Source: CAD feature listing. Evaluate the final solid. Frame: model axes, mm. Coordinates: 2 decimals unless noted, no trailing zeros. Order: outer loops, then holes, each group sorted by start corner. A loop starts at its lowest first (then second) coordinate and runs counter-clockwise, first axis right, second up.
Item 1: Section A-A on z = 0. Return the cut outline in (x, y), then the cut area to 3 significant figures.
Item 2: Ray query, line 1 (Y direction, x = 132.7, z = 0); line 2 (Z direction, x = 134.5, y = 16.25); line 3 (Z direction, x = 133.85, y = -21.1). Return the intervals inside material, ascending.
Item 3: Mould query, pull axis Y, two halves, no side actions, for faces 1 (the flat face through (131.7, 20, -20)), 2 (the cylindrical face through (133.672, -30.864, 0.215)), 3 (the cylindrical face through (133.73, -45.61, -5.99)). Classes: released by +Y, released by -Y, zero draft, split by the parting line, or undercut.
Item 4: Section B-B on y = 0. Return the cut outline in (x, z).
Item 5: Section C-C on x = 133.2. Return the cut outline in (y, z), then the cut area to 3 significant figures.
Item 6: Contact query for flat-ended pins moving along their axis: P1, Ø2.5, axis at y = 16.25, z = -28.15, coming from the -X side; P2, Ø1, axis at x = 132, y = 7, coming from the -Z side; P3, Ø2, axis at x = 132, z = -19, coming from the -Y side; P4, Ø1.5, axis at x = 133.5, z = -9, coming from the +Y side. Output: stop coordinate, or through.
Item 7: Section D-D on y = -21.1. Return the cut outline in (x, z), then the cut area to 3 significant figures.
from build123d import *

# Parameters (mm, degrees)
AXIAL_PROFILE_MM_W     = 4
AXIAL_PROFILE_MM_H     = 19
AXIAL_HOLES_DEPTH      = 151.487507787
AXIAL_HOLES_DEPTH_BACK = 151.487507787
SKETCH2_R              = 1.65


with BuildPart() as part:
    # Axial profile (mm) → Full revolution (revolve)
    with BuildSketch(Plane.XY, mode=Mode.PRIVATE) as full_revolution_sk:
        with Locations((133.7, 36.5)):
            Rectangle(AXIAL_PROFILE_MM_W, AXIAL_PROFILE_MM_H)
    revolve(full_revolution_sk.sketch.rotate(Axis((-110, 0, 0), (1, 0, 0)), 90), axis=Axis((-110, 0, 0), (1, 0, 0)))

    # Sketch2 → Axial holes (cut, two sides: drawn at the far end of the back side and taken through both)
    with BuildSketch(Plane(origin=(0, 0, 0), x_dir=(0, 0, -1), z_dir=(1, 0, 0)).offset(-AXIAL_HOLES_DEPTH_BACK)):
        with Locations((0, 42.2)):
            Circle(SKETCH2_R)
        with Locations((-36.54627204, -21.1)):
            Circle(SKETCH2_R)
        with Locations((36.54627204, -21.1)):
            Circle(SKETCH2_R)
        with Locations((-28.145825623, 16.25)):
            Circle(SKETCH2_R)
        with Locations((0, -32.5)):
            Circle(SKETCH2_R)
        with Locations((28.145825623, 16.25)):
            Circle(SKETCH2_R)
    extrude(amount=AXIAL_HOLES_DEPTH + AXIAL_HOLES_DEPTH_BACK, mode=Mode.SUBTRACT)


solid = part.part
Answer list:
1. outline: (131.7, -46) - (135.7, -46) - (135.7, -34.15) - (131.7, -34.15) - close; (131.7, -30.85) - (135.7, -30.85) - (135.7, -27) - (131.7, -27) - close; (131.7, 27) - (135.7, 27) - (135.7, 40.55) - (131.7, 40.55) - close; (131.7, 43.85) - (135.7, 43.85) - (135.7, 46) - (131.7, 46) - close
1. area: 126 mm2
2. line 1: y = -46 to -34.15, -30.85 to -27, 27 to 40.55, 43.85 to 46
2. line 2: z = -43.03 to -29.8, -26.5 to -21.56, 21.56 to 26.5, 29.8 to 43.03
2. line 3: z = -40.88 to -38.2, -34.9 to -16.85, 16.85 to 34.9, 38.2 to 40.88
3. face 1: zero draft
3. face 2: undercut
3. face 3: split by the parting line
4. outline: (131.7, -46) - (135.7, -46) - (135.7, -27) - (131.7, -27) - close; (131.7, 27) - (135.7, 27) - (135.7, 46) - (131.7, 46) - close
5. outline: circle Ø92 at (0, 0); hole circle Ø3.3 at (-32.5, 0); hole circle Ø54 at (0, 0); hole circle Ø3.3 at (-21.1, -36.55); hole circle Ø3.3 at (-21.1, 36.55); hole circle Ø3.3 at (16.25, -28.15); hole circle Ø3.3 at (16.25, 28.15); hole circle Ø3.3 at (42.2, 0)
5. area: 4,310 mm2
6. P1: passes through
6. P2: stops at z = -45.54
6. P3: stops at y = -42.33
6. P4: stops at y = 45.25
7. outline: (131.7, -40.88) - (135.7, -40.88) - (135.7, -38.2) - (131.7, -38.2) - close; (131.7, -34.9) - (135.7, -34.9) - (135.7, -16.85) - (131.7, -16.85) - close; (131.7, 16.85) - (135.7, 16.85) - (135.7, 34.9) - (131.7, 34.9) - close; (131.7, 38.2) - (135.7, 38.2) - (135.7, 40.88) - (131.7, 40.88) - close
7. area: 166 mm2
